from build123d import *

# Parameters (mm, degrees)
ESQUISSE1_W             = 39
ESQUISSE1_H             = 62
BOSS_EXTRU_1_DEPTH      = 10
ESQUISSE2_R             = 4
ENL_V_MAT_EXTRU_1_DEPTH = 10
CONG_1_R                = 10
BOSS_EXTRU_2_DEPTH      = 80
CONG_2_R                = 10
ESQUISSE4_W             = 39
ESQUISSE4_H             = 62
BOSS_EXTRU_3_DEPTH      = 10
CONG_3_START            = 10
CONG_3_DEPTH            = 91
ENL_V_START             = -100
ESQUISSE5_R             = 4
ENL_V_MAT_EXTRU_2_DEPTH = 100
ESQUISSE6_W             = 39
ESQUISSE6_H             = 5
BOSS_EXTRU_4_DEPTH      = 80
ESQUISSE7_R             = 11.5
ENL_V_MAT_EXTRU_3_DEPTH = 112.722871427


with BuildPart() as part:
    # Esquisse1 → Boss.-Extru.1 (new body)
    with BuildSketch(Plane.XY):
        Rectangle(ESQUISSE1_W, ESQUISSE1_H)
    extrude(amount=BOSS_EXTRU_1_DEPTH)

    # Esquisse2 → Enlèv. mat.-Extru.1 (cut)
    with BuildSketch(Plane.XY.offset(10)):
        with Locations((0, 21)):
            Circle(ESQUISSE2_R)
        with Locations((0, -21)):
            Circle(ESQUISSE2_R)
    extrude(amount=-ENL_V_MAT_EXTRU_1_DEPTH, mode=Mode.SUBTRACT)

    # Congé1
    cong_1_edges = [part.edges().sort_by_distance(p)[0] for p in [
        (-19.5, 31, 5),
        (-19.5, -31, 5),
        (19.5, -31, 5),
        (19.5, 31, 5),
    ]]
    fillet(cong_1_edges, radius=CONG_1_R)

    # Esquisse3 → Boss.-Extru.2 (add)
    with BuildSketch(Plane.XY.offset(10)):
        Polygon((0, 25), (19.5, 25), (19.5, 31), (-19.5, 31), (-19.5, 25), align=None)
        Polygon((0, -25), (19.5, -25), (19.5, -31), (-19.5, -31), (-19.5, -25), align=None)
    extrude(amount=BOSS_EXTRU_2_DEPTH)

    # Congé2
    # the kernel refuses this fillet: 10 mm, written as the material it takes off along each edge
    with BuildSketch(Plane(origin=(-19.5, 31, -12.912878475), x_dir=(1, 0, 0), z_dir=(0, 0, 1)), Plane(origin=(19.5, -31, -12.912878475), x_dir=(-1, 0, 0), z_dir=(0, 0, 1))) as cong_2_piece_1:
        with BuildLine():
            CenterArc((9.16515139, -10), CONG_2_R, 90, 66.421821522)
            Line((0, -6), (-0.183303028, -5.92))
            ThreePointArc((-0.183303028, -5.92), (-0.2, -3), (-0.2, 0))
            Line((-0.2, 0), (0, 0.2))
            Line((0, 0.2), (9.16515139, 0.2))
            Line((9.16515139, 0.2), (9.16515139, 0))
        make_face()
    extrude(amount=125.82575695, mode=Mode.SUBTRACT)
    with BuildSketch(Plane(origin=(19.5, 31, -12.912878475), x_dir=(-1, 0, 0), z_dir=(0, 0, 1)), Plane(origin=(-19.5, -31, -12.912878475), x_dir=(1, 0, 0), z_dir=(0, 0, 1))) as cong_2_piece_2:
        with BuildLine():
            CenterArc((9.16515139, 10), CONG_2_R, 203.578178478, 66.421821522)
            Line((0, 6), (-0.183303028, 5.92))
            ThreePointArc((-0.183303028, 5.92), (-0.2, 3), (-0.2, 0))
            Line((-0.2, 0), (0, -0.2))
            Line((0, -0.2), (9.16515139, -0.2))
            Line((9.16515139, -0.2), (9.16515139, 0))
        make_face()
    extrude(amount=125.82575695, mode=Mode.SUBTRACT)

    # Esquisse4 → Boss.-Extru.3 (add)
    with BuildSketch(Plane.XY.offset(90)):
        Rectangle(ESQUISSE4_W, ESQUISSE4_H)
    extrude(amount=BOSS_EXTRU_3_DEPTH)

    # Congé3: read off the stored shape, not the designer's step
    # Congé3 outline → Congé3 (cut)
    with BuildSketch(Plane.XY.offset(CONG_3_START)):
        with BuildLine():
            ThreePointArc((-9.5, -31), (-16.571067812, -28.071067812), (-19.5, -21))
            Line((-19.5, -21), (-19.5, -31))
            Line((-19.5, -31), (-9.5, -31))
        make_face()
        with BuildLine():
            ThreePointArc((19.5, -21), (16.571067812, -28.071067812), (9.5, -31))
            Line((9.5, -31), (19.5, -31))
            Line((19.5, -31), (19.5, -21))
        make_face()
        with BuildLine():
            ThreePointArc((-19.5, 21), (-16.571067812, 28.071067812), (-9.5, 31))
            Line((-9.5, 31), (-19.5, 31))
            Line((-19.5, 31), (-19.5, 21))
        make_face()
        with BuildLine():
            ThreePointArc((9.5, 31), (16.571067812, 28.071067812), (19.5, 21))
            Line((19.5, 21), (19.5, 31))
            Line((19.5, 31), (9.5, 31))
        make_face()
    extrude(amount=CONG_3_DEPTH, mode=Mode.SUBTRACT)

    # Esquisse5 → Enlèv. mat.-Extru.2 (cut)
    with BuildSketch(Plane(origin=(0, 0, 90), x_dir=(-1, 0, 0), z_dir=(0, 0, -1)).offset(ENL_V_START)):
        with Locations(Location((0, 21, 0), (0, 0, 180))):
            Circle(ESQUISSE5_R)
        with Locations(Location((0, -21, 0), (0, 0, 180))):
            Circle(ESQUISSE5_R)
    extrude(amount=ENL_V_MAT_EXTRU_2_DEPTH, mode=Mode.SUBTRACT)

    # Esquisse6 → Boss.-Extru.4 (add)
    with BuildSketch(Plane(origin=(0, 0, 90), x_dir=(-1, 0, 0), z_dir=(0, 0, -1))):
        with Locations((0, -14)):
            Rectangle(ESQUISSE6_W, ESQUISSE6_H)
    extrude(amount=BOSS_EXTRU_4_DEPTH)

    # Esquisse7 → Enlèv. mat.-Extru.3 (cut, through all)
    with BuildSketch(Plane.ZY.offset(19.5)):
        with Locations((50, -3.5)):
            Circle(ESQUISSE7_R)
    extrude(amount=-ENL_V_MAT_EXTRU_3_DEPTH, mode=Mode.SUBTRACT)


solid = part.part
Verification items for the finished model (mm, model axes). A direction names the side the tool comes from. Coordinates: 2 decimals unless noted, no trailing zeros. Write each loop counter-clockwise with the first axis right and the second up, starting at its lowest first coordinate (ties: lowest second). Pieces come first, ordered by that corner, then holes. Notation, with made-up numbers: M -32,34 L -18,34 A17 ccw -18,56 Z; hole C -6.5,27 d3. An arc over 180 degrees is marked long. Use a Markdown table: item, result.
Q1. Set-up check for faces 1 (the face through (0, -16.5, 51)), 2 (the face through (19.5, -13, 57)): record each of +Z, -Z, +X, -X, +Y, -Y from which the full face is reachable in a straight line by a thin tool's end or side.
Reply:
| item | result |
|---|---|
| face 1 | +X, -X |
| face 2 | +Z, -Z, +X, +Y, -Y |
Q2. Sectioned sample at B-B, the plane z = 28. Record the boundary of the cut face in (x, y).
Reply:
| item | result |
|---|---|
| outline | M -19.5,-16.5 L 19.5,-16.5 L 19.5,-11.5 L -19.5,-11.5 Z; M -18.67,-25 A10 ccw -9.5,-31 L 9.5,-31 A10 ccw 18.67,-25 Z; M -18.67,25 L 18.67,25 A10 ccw 9.5,31 L -9.5,31 A10 ccw Z |
Q3. Thickness scan on line 1 (Y direction, x = 0, z = 2.75); line 2 (Y direction, x = 10, z = 10.5); line 3 (X direction, y = -21, z = 2). Record the ranges inside material, lowest first.
Reply:
| item | result |
|---|---|
| line 1 | y = -31 to -25, -17 to 17, 25 to 31 |
| line 2 | y = -30.99 to -25, -16.5 to -11.5, 25 to 30.99 |
| line 3 | x = -19.5 to -4, 4 to 19.5 |
Q4. Draft check along Z on faces 3 (the face through (-0.521, 17.034, 95.07)), 4 (the face through (0, 0, 100)), 5 (the face through (0, -11.5, 74)). Enter one of: +Z half, -Z half, draft (parallel to the pull), parting line (faces both ways), or undercut.
Reply:
| item | result |
|---|---|
| face 3 | draft |
| face 4 | +Z half |
| face 5 | undercut |
Q5. Go/stop test with flat-tipped pins: P1, Ø5, axis at x = 0, y = 21, coming from the -Z side; P2, Ø1.5, axis at x = -11.5, z = 56.5, coming from the +Y side; P3, Ø4, axis at x = 11.5, y = -11.5, coming from the -Z side. Record where each tip stops, or that it passes through.
Reply:
| item | result |
|---|---|
| P1 | passes through |
| P2 | stops at y = 30.92 |
| P3 | stops at z = 0 |
Q6. Sectioned sample at A-A, the plane y = 8. Record the boundary of the cut face in (x, z).
Reply:
| item | result |
|---|---|
| outline | M -19.5,0 L 19.5,0 L 19.5,10 L -19.5,10 Z; M -19.5,90 L 19.5,90 L 19.5,100 L -19.5,100 Z |
Q7. Sectioned sample at C-C, the plane x = -5. Record the boundary of the cut face in (y, z).
Reply:
| item | result |
|---|---|
| outline | M -31,0 L 31,0 L 31,100 L -31,100 Z; hole M -25,10 L -16.5,10 L -16.5,90 L -25,90 Z; hole M -11.5,10 L 25,10 L 25,90 L -11.5,90 L -11.5,58.26 A11.5 ccw -11.5,41.74 Z |
Q8. Sectioned sample at D-D, the plane y = 24. Record the boundary of the cut face in (x, z).
Reply:
| item | result |
|---|---|
| outline | M -19.04,0 L -2.65,0 L -2.65,10 L -19.04,10 Z; M -19.04,90 L -2.65,90 L -2.65,100 L -19.04,100 Z; M 2.65,0 L 19.04,0 L 19.04,10 L 2.65,10 Z; M 2.65,90 L 19.04,90 L 19.04,100 L 2.65,100 Z |
